```python
from build123d import *

# Parameters (mm, degrees)
SKETCH1_R           = 3
BOSS_EXTRUDE1_DEPTH = 10
SKETCH2_R           = 1.957866775
CUT_EXTRUDE1_DEPTH  = 1
SKETCH3_W           = 6
SKETCH3_H           = 1.413467244
BOSS_EXTRUDE2_DEPTH = 3
SKETCH4_W           = 1.123078493
SKETCH4_H           = 2.580406537
BOSS_EXTRUDE3_DEPTH = 0.5


with BuildPart() as part:
    # Sketch1 → Boss-Extrude1 (new body)
    with BuildSketch(Plane(origin=(0, 0, 0), x_dir=(0, 0, -1), z_dir=(1, 0, 0))):
        Circle(SKETCH1_R)
    extrude(amount=BOSS_EXTRUDE1_DEPTH)

    # Sketch2 → Cut-Extrude1 (cut)
    with BuildSketch(Plane(origin=(10, 0, 0), x_dir=(0, 0, -1), z_dir=(1, 0, 0))):
        Circle(SKETCH2_R)
    extrude(amount=-CUT_EXTRUDE1_DEPTH, mode=Mode.SUBTRACT)

    # Sketch3 → Boss-Extrude2 (add)
    with BuildSketch(Plane.ZY):
        Rectangle(SKETCH3_W, SKETCH3_H)
    extrude(amount=BOSS_EXTRUDE2_DEPTH)

    # Sketch4 → Boss-Extrude3 (add)
    with BuildSketch(Plane(origin=(0, 0.706733622, 0), x_dir=(1, 0, 0), z_dir=(0, 1, 0))):
        with Locations((-1.88810277, 0.401099462)):
            Rectangle(SKETCH4_W, SKETCH4_H)
    extrude(amount=BOSS_EXTRUDE3_DEPTH)


solid = part.part
```
Check sheet for the modelled part. Datum: model origin and axes. Units: mm. A direction names the side the tool comes from. Round coordinates to 2 decimals unless told otherwise and drop trailing zeros. Loops run counter-clockwise (first coordinate to the right, second up) from the corner with the lowest first, then second, coordinate; pieces in that order, holes last. Notation, with made-up numbers: (13.25, -31) - (23.25, -31) arc R33 cw to (23.25, 4) - close; hole circle Ø7 at (36, 50.5). An arc over 180 degrees is marked (long way). Answer as a JSON object with one key per item and string values. Group by question number.
Q1. Set-up check for faces 1 (the face through (-1, -0.707, 0)), 2 (the face through (9, 0, 0)), 3 (the face through (0, 2, 0)), 4 (the face through (-2, 1.207, 0)): record each of +Z, -Z, +X, -X, +Y, -Y from which the full face is reachable in a straight line by a thin tool's end or side.
Q2. Sectioned sample at A-A, the plane x = -1.5. Enter the section's corners in (y, z).
Q3. Scan lines: line 1 along Y through (x, z) = (9.35, 0); line 2 along Y through (x, z) = (0.5, -0.7). Record each from-to range of solid material in increasing order. Write a range as [from, to].
Q4. Gauge pin test, flat ends, axial feed: P1, Ø2.5, axis at y = 2, z = -1, coming from the -X side; P2, Ø3.5, axis at x = -2, z = -0.5, coming from the +Y side; P3, Ø1.5, axis at x = 1.5, z = 1, coming from the +Y side; P4, Ø2.5, axis at y = -1.5, z = 1, coming from the -X side. Record the tip position at first contact, or that the pin passes through.
Q5. Mould release check, pull along X, two halves, no side actions. Record for faces 5 (the face through (-1, 0.707, 0)), 6 (the face through (10, -2, -1)), 7 (the face through (5, 0, 3)): released by +X, released by -X, zero draft, split by the parting line, or undercut.
Q6. Sectioned sample at D-D, the plane z = 1.35. Enter the section's corners in (x, y).
Q7. Sectioned sample at B-B, the plane z = 0. Enter the section's corners in (x, y).
Q8. Sectioned sample at C-C, the plane y = -1.3. Enter the section's corners in (x, z), plus the area to 3 significant figures.
Solution:
{
 "1": {"face 1": "+Z, -Z, -X, -Y", "face 2": "+X", "face 3": "+Z, -Z, +Y", "face 4": "+Z, -Z, -X, +Y"},
 "2": {"outline": "(-0.71, -3) - (0.71, -3) - (0.71, -1.69) - (1.21, -1.69) - (1.21, 0.89) - (0.71, 0.89) - (0.71, 3) - (-0.71, 3) - close"},
 "3": {"line 1": "y = [-3, -1.96], [1.96, 3]", "line 2": "y = [-2.92, 2.92]"},
 "4": {"P1": "stops at x = -2.45", "P2": "stops at y = 1.21", "P3": "stops at y = 2.99", "P4": "stops at x = -3"},
 "5": {"face 5": "undercut", "face 6": "released by +X", "face 7": "zero draft"},
 "6": {"outline": "(-3, -0.71) - (0, -0.71) - (0, -2.68) - (10, -2.68) - (10, -1.42) - (9, -1.42) - (9, 1.42) - (10, 1.42) - (10, 2.68) - (0, 2.68) - (0, 0.71) - (-3, 0.71) - close"},
 "7": {"outline": "(-3, -0.71) - (0, -0.71) - (0, -3) - (10, -3) - (10, -1.96) - (9, -1.96) - (9, 1.96) - (10, 1.96) - (10, 3) - (0, 3) - (0, 0.71) - (-1.33, 0.71) - (-1.33, 1.21) - (-2.45, 1.21) - (-2.45, 0.71) - (-3, 0.71) - close"},
 "8": {"outline": "(0, -2.7) - (10, -2.7) - (10, -1.46) - (9, -1.46) - (9, 1.46) - (10, 1.46) - (10, 2.7) - (0, 2.7) - close", "area": "51.1 mm²"}
}
